from build123d import *

# Parameters (mm, degrees)
CYLINDER070_R     = 1.6
CYLINDER070_DEPTH = 100
BOX031_W          = 50
BOX031_H          = 19.558
BOX031_DEPTH      = 19.558
BOX030_W          = 38
BOX030_H          = 35
BOX030_DEPTH      = 35
FILLET006_R       = 5
FILLET007_R       = 3


with BuildPart() as cylinder070:
    # Cylinder070 → Cylinder070 (new body)
    with BuildSketch(Plane(origin=(543.2, 13.75, 60), x_dir=(1, 0, 0), z_dir=(0, 0, 1))):
        Circle(CYLINDER070_R)
    extrude(amount=CYLINDER070_DEPTH)


with BuildPart() as cube031:
    # Box031 → Box031 (new body)
    with BuildSketch(Plane(origin=(528.17, -9.779, 103.467), x_dir=(1, 0, 0), z_dir=(0, 0, 1))):
        with Locations((25, 9.779)):
            Rectangle(BOX031_W, BOX031_H)
    extrude(amount=BOX031_DEPTH)


with BuildPart() as cut039:
    # Box030 → Box030 (new body)
    with BuildSketch(Plane(origin=(534.67, -17.5, 95.25), x_dir=(1, 0, 0), z_dir=(0, 0, 1))):
        with Locations((19, 17.5)):
            Rectangle(BOX030_W, BOX030_H)
    extrude(amount=BOX030_DEPTH)

    # Cut038: cut Cube031
    add(cube031.part, mode=Mode.SUBTRACT)


with BuildPart() as cut039_1:
    # Cut038 placement: moved
    add(cut039.part.moved(Location((-10.3, 0, -16.6))))

    # Fillet006
    fillet006_edges = [cut039_1.edges().sort_by_distance(p)[0] for p in [
        (543.37, -17.5, 78.65),
        (543.37, -17.5, 113.65),
        (543.37, 17.5, 113.65),
        (543.37, 17.5, 78.65),
    ]]
    fillet(fillet006_edges, radius=FILLET006_R)

    # Fillet007
    fillet007_edges = [cut039_1.edges().sort_by_distance(p)[0] for p in [
        (524.37, 0, 78.65),
        (562.37, 0, 78.65),
    ]]
    fillet(fillet007_edges, radius=FILLET007_R)

    # Cut039: cut Cylinder070
    add(cylinder070.part, mode=Mode.SUBTRACT)


solid = cut039_1.part
CAD build for the part. Positions are in the model's coordinates, mm. A direction names the side the tool comes from. Round coordinates to 2 decimals unless told otherwise and drop trailing zeros. Loops run counter-clockwise (first coordinate to the right, second up) from the corner with the lowest first, then second, coordinate; pieces in that order, holes last. Notation, with made-up numbers: (17, 65) - (65, 65) arc R24 ccw to (65, 102) - close; hole circle Ø1 at (-10.75, 77.5). An arc over 180 degrees is marked (long way). Put each result on its own line as item: value.
1. Slice it at D-D on x = 543.2. List the corners of the cut face in (y, z) (3 decimals).
Geometry check:
outline: (-17.5, 83.65) arc R5 ccw to (-12.5, 78.65) - (12.15, 78.65) - (12.15, 113.65) - (-12.5, 113.65) arc R5 ccw to (-17.5, 108.65) - close; (15.35, 79.542) arc R5 ccw to (17.5, 83.65) - (17.5, 108.65) arc R5 ccw to (15.35, 112.758) - close; hole (-9.779, 86.867) - (9.779, 86.867) - (9.779, 106.425) - (-9.779, 106.425) - close
2. Two-plate mould, pull along X, no slides. Class faces 3 (the cylindrical face through (561.47, 16.64, 96.32)), 4 (the cylindrical face through (525.23, 16.6, 96.32)), 5 (the cylindrical face through (541.6, 13.8, 95.9)), 6 (the flat face through (543, 9.779, 97)): released by +X, released by -X, zero draft, split by the parting line, or undercut.
Geometry check:
face 3: released by +X
face 4: released by -X
face 5: undercut
face 6: zero draft
3. Slice it at C-C on y = 0. List the corners of the cut face in (x, z) (3 decimals).
Geometry check:
outline: (524.37, 81.65) arc R3 ccw to (527.37, 78.65) - (559.37, 78.65) arc R3 ccw to (562.37, 81.65) - (562.37, 86.867) - (524.37, 86.867) - close; (524.37, 106.425) - (562.37, 106.425) - (562.37, 110.65) arc R3 ccw to (559.37, 113.65) - (527.37, 113.65) arc R3 ccw to (524.37, 110.65) - close
4. Slice it at B-B on x = 534. List the corners of the cut face in (y, z) (3 decimals).
Geometry check:
outline: (-17.5, 83.65) arc R5 ccw to (-12.5, 78.65) - (12.5, 78.65) arc R5 ccw to (17.5, 83.65) - (17.5, 108.65) arc R5 ccw to (12.5, 113.65) - (-12.5, 113.65) arc R5 ccw to (-17.5, 108.65) - close; hole (-9.779, 86.867) - (9.779, 86.867) - (9.779, 106.425) - (-9.779, 106.425) - close
5. Slice it at A-A on z = 97.5. List the corners of the cut face in (x, y).
Geometry check:
outline: (524.37, -14.5) arc R3 ccw to (527.37, -17.5) - (559.37, -17.5) arc R3 ccw to (562.37, -14.5) - (562.37, -9.78) - (524.37, -9.78) - close; (524.37, 9.78) - (562.37, 9.78) - (562.37, 14.5) arc R3 ccw to (559.37, 17.5) - (527.37, 17.5) arc R3 ccw to (524.37, 14.5) - close; hole circle Ø3.2 at (543.2, 13.75)
6. 3-axis set-ups, long thin cutter, end or side, ignore diameter. For faces 1 (the cylindrical face through (543.59, 16, 112.22)), 2 (the flat face through (543, 0, 106.425)): which of +Z, -Z, +X, -X, +Y, -Y reach the whole face in a straight line?
Geometry check:
face 1: +Z, +X, -X, +Y
face 2: +X, -X
7. Wall check: line 1 (Y direction, x = 543, z = 95); line 2 (Z direction, x = 528.5, y = 8) (3 decimals); line 3 (Y direction, x = 558, z = 103). Give the ranges that are in metal, low to high.
Geometry check:
line 1: -17.5 to -9.78, 9.78 to 12.16, 15.34 to 17.5
line 2: 78.65 to 86.867, 106.425 to 113.65
line 3: -17.5 to -9.78, 9.78 to 17.5
